Source: CAD feature listing. Evaluate the final solid. Frame: model axes, mm. Round coordinates to 2 decimals unless told otherwise and drop trailing zeros. Loops run counter-clockwise (first coordinate to the right, second up) from the corner with the lowest first, then second, coordinate; pieces in that order, holes last. Notation, with made-up numbers: M 55,89 L 106,89 A7 cw 106,97 Z; hole C 8,-8.5 d10. An arc over 180 degrees is marked long. One line per item, written item: value.
from build123d import *

# Parameters (mm, degrees)
F0_R     = 485
F1_DEPTH = 35
F2_D     = 6.6
F2_DEPTH = 19.75
F2_TIP   = 1.9828400428


with BuildPart() as f1:
    # F0 (on Front) → F1 (new body)
    with BuildSketch(Plane.XZ):
        Circle(F0_R)
    extrude(amount=-F1_DEPTH)

    # F2
    with Locations(Plane.XZ):
        with Locations((-325, 0), (-320.062519729, 56.4356577418), (-305.4001017554, 111.1565465808), (-281.4582562299, 162.5), (-248.9644440137, 208.9059731481), (-208.9059731481, 248.9644440137), (-162.5, 281.4582562299), (-111.1565465808, 305.4001017554), (-56.4356577418, 320.062519729), (0, 325), (0, 425), (-73.8004755084, 418.5432950302), (-145.3585609134, 399.369363834), (-212.5, 368.0607966084), (-273.1847341168, 325.5688883256), (-325.5688883256, 273.1847341168), (-368.0607966084, 212.5), (-399.369363834, 145.3585609134), (-418.5432950302, 73.8004755084), (-425, 0)):
            Hole(F2_D / 2, depth=F2_DEPTH)
            with Locations((0, 0, -(F2_DEPTH + F2_TIP / 2))):  # 118° drill point
                Cone(0, F2_D / 2, F2_TIP, mode=Mode.SUBTRACT)


solid = f1.part
1. Ray query, line 1 (X direction, y = 2, z = 2); line 2 (Z direction, x = -273.5, y = 17); line 3 (Z direction, x = -425, y = 4.25). Return the intervals inside material, ascending. Write a range as [from, to].
Report:
line 1: x = [-485, -427.62], [-422.38, -327.62], [-322.38, 485]
line 2: z = [-400.53, 322.28], [328.85, 400.53]
line 3: z = [-233.67, -3.3], [3.3, 233.67]
2. Section query A-A (x = 410). Return the cut outline in (y, z), and give its area (3 significant figures).
Report:
outline: M 0,-259.08 L 35,-259.08 L 35,259.08 L 0,259.08 Z
area: 18,100 mm2
3. Section query B-B (z = -169). Return the cut outline in (x, y).
Report:
outline: M -454.6,0 L 454.6,0 L 454.6,35 L -454.6,35 Z
4. Pin query (flat end, axial travel): pin 1 (8 mm diameter, centred on x = 123, y = 4.5, fed in from -Z); pin 2 (5.5 mm diameter, centred on x = -111.16, z = 305.4, fed in from -Y); pin 3 (1.5 mm diameter, centred on x = 51.5, y = 5, fed in from -Z). Return the tip coordinate at first contact, or that it passes through.
Report:
pin 1: stops at z = -470.17
pin 2: stops at y = 20.08
pin 3: stops at z = -482.34
